```python
from build123d import *

# Parameters (mm, degrees)
CROQUIS1_R              = 10.5
SALIENTE_EXTRUIR1_DEPTH = 2.5
CROQUIS2_R              = 4.5
CROQUIS2_R_2            = 3
SALIENTE_EXTRUIR2_DEPTH = 3
CROQUIS4_R              = 4.75
CROQUIS4_R_2            = 3.25
CORTAR_EXTRUIR1_DEPTH   = 1
CROQUIS5_R              = 3
CORTAR_EXTRUIR2_DEPTH   = 1
CROQUIS6_R              = 1.5
CORTAR_EXTRUIR3_DEPTH   = 3
CROQUIS7_R              = 1
CORTAR_EXTRUIR4_DEPTH   = 3


with BuildPart() as part:
    # Croquis1 → Saliente-Extruir1 (new body)
    with BuildSketch(Plane(origin=(0, 0, 0), x_dir=(1, 0, 0), z_dir=(0, 1, 0))):
        with Locations(Location((0, 0, 0), (0, 0, 270))):
            Circle(CROQUIS1_R)
    extrude(amount=SALIENTE_EXTRUIR1_DEPTH)

    # Croquis2 → Saliente-Extruir2 (add)
    with BuildSketch(Plane(origin=(0, 2.5, 0), x_dir=(1, 0, 0), z_dir=(0, 1, 0))):
        with Locations(Location((0, 0, 0), (0, 0, 270))):
            Circle(CROQUIS2_R)
        with Locations(Location((0, 0, 0), (0, 0, 270))):
            Circle(CROQUIS2_R_2, mode=Mode.SUBTRACT)
    extrude(amount=SALIENTE_EXTRUIR2_DEPTH)

    # Croquis4 → Cortar-Extruir1 (cut)
    with BuildSketch(Plane.XZ):
        with Locations(Location((0, 0, 0), (0, 0, 270))):
            Circle(CROQUIS4_R)
        with Locations(Location((0, 0, 0), (0, 0, 270))):
            Circle(CROQUIS4_R_2, mode=Mode.SUBTRACT)
    extrude(amount=-CORTAR_EXTRUIR1_DEPTH, mode=Mode.SUBTRACT)

    # Croquis5 → Cortar-Extruir2 (cut)
    with BuildSketch(Plane.XZ):
        with Locations(Location((0, 0, 0), (0, 0, 90))):
            Circle(CROQUIS5_R)
    extrude(amount=-CORTAR_EXTRUIR2_DEPTH, mode=Mode.SUBTRACT)

    # Croquis6 → Cortar-Extruir3 (cut)
    with BuildSketch(Plane.XZ.offset(-1)):
        with Locations(Location((0, 0, 0), (0, 0, 270))):
            Circle(CROQUIS6_R)
    extrude(amount=-CORTAR_EXTRUIR3_DEPTH, mode=Mode.SUBTRACT)

    # Croquis7 → Cortar-Extruir4 (cut)
    with BuildSketch(Plane.XZ):
        with Locations(Location((0, 7.2, 0), (0, 0, 270))):
            Circle(CROQUIS7_R)
        with Locations(Location((0, -7.2, 0), (0, 0, 90))):
            Circle(CROQUIS7_R)
        with Locations(Location((7.2, 0, 0), (0, 0, 270))):
            Circle(CROQUIS7_R)
        with Locations(Location((-7.2, 0, 0), (0, 0, 90))):
            Circle(CROQUIS7_R)
        with Locations(Location((3.5, 7.2, 0), (0, 0, 270))):
            Circle(CROQUIS7_R)
        with Locations(Location((-3.5, 7.2, 0), (0, 0, 270))):
            Circle(CROQUIS7_R)
        with Locations(Location((3.5, -7.2, 0), (0, 0, 90))):
            Circle(CROQUIS7_R)
        with Locations(Location((-3.5, -7.2, 0), (0, 0, 90))):
            Circle(CROQUIS7_R)
        with Locations(Location((7.2, 3, 0), (0, 0, 270))):
            Circle(CROQUIS7_R)
        with Locations(Location((7.2, -3, 0), (0, 0, 270))):
            Circle(CROQUIS7_R)
        with Locations(Location((-7.2, -3, 0), (0, 0, 90))):
            Circle(CROQUIS7_R)
        with Locations(Location((-7.2, 3, 0), (0, 0, 90))):
            Circle(CROQUIS7_R)
    extrude(amount=-CORTAR_EXTRUIR4_DEPTH, mode=Mode.SUBTRACT)


solid = part.part
```
Read the model definition and answer for the solid it produces. Units are mm, in the model's axes. A direction names the side the tool comes from. Coordinates: 2 decimals unless noted, no trailing zeros. Write each loop counter-clockwise with the first axis right and the second up, starting at its lowest first coordinate (ties: lowest second). Pieces come first, ordered by that corner, then holes. Notation, with made-up numbers: (84, 49.25) -> (116, 49.25) arc R28 ccw to (116, 81.25) -> close; hole circle Ø1 at (28.25, 64.25). An arc over 180 degrees is marked (long way). Return JSON: item names as keys, results as strings.
1. A cutting plane is placed at A-A (y = 0.3). Give the number of separate pieces and of enclosed holes in the cut face, and give its area (3 significant figures).
Found:
{"separate pieces": "2", "enclosed holes": "14", "area": "243 mm2"}
2. Determine the mould class of faces 4 (the face through (-3, 1, -2)), 5 (the face through (-8.04, 1.23, 0.54)), 6 (the face through (3.2, 1.2, 10)), 7 (the face through (-2, 0, 5)) for opening direction X: pulls with the +X half, pulls with the -X half, needs draft (parallel to the pull), parting line crosses it, or undercut.
Found:
{"face 4": "undercut", "face 5": "undercut", "face 6": "parting line crosses it", "face 7": "needs draft"}
3. A cutting plane is placed at D-D (z = -7). Determine the outline of the cut face in (x, y).
Found:
{"outline": "(-7.83, 0) -> (-4.48, 0) -> (-4.48, 2.5) -> (-7.83, 2.5) -> close; (-2.52, 0) -> (-0.98, 0) -> (-0.98, 2.5) -> (-2.52, 2.5) -> close; (0.98, 0) -> (2.52, 0) -> (2.52, 2.5) -> (0.98, 2.5) -> close; (4.48, 0) -> (7.83, 0) -> (7.83, 2.5) -> (4.48, 2.5) -> close"}
4. Each of these flat-tipped pins is pushed along its axis until it touches: P1, Ø2.5, axis at x = 0, z = 0, coming from the +Y side; P2, Ø2.5, axis at x = -7.2, z = 3, coming from the +Y side; P3, Ø2, axis at y = 3, z = 7.5, coming from the +X side; P4, Ø1.8, axis at x = 0.5, z = 0.5, coming from the -Y side. Where does it stop, or does it pass through?
Found:
{"P1": "through", "P2": "y = 2.5", "P3": "x = 8.14", "P4": "y = 1"}
5. Find the intervals of material crossed by line 1 along X through (y, z) = (0.95, 0); line 2 along Z through (x, y) = (4, 0.65); line 3 along X through (y, z) = (0.5, 7.2), in increasing order. Write a range as from..to.
Found:
{"line 1": "-10.5..-8.2, -6.2..-4.75, -3.25..-3, 3..3.25, 4.75..6.2, 8.2..10.5", "line 2": "-9.71..-8.07, -6.33..-2.56, 2.56..6.33, 8.07..9.71", "line 3": "-7.64..-4.5, -2.5..-1, 1..2.5, 4.5..7.64"}
6. A tool of negligible diameter and unlimited length cuts with its end or side. For faces 1 (the face through (-1.3, 2.5, 1.3)), 2 (the face through (-0.383, 1.232, 6.276)), 3 (the face through (-1.978, 0.493, 2.579)), from which of +Z, -Z, +X, -X, +Y, -Y can it reach the whole face along a straight path? Write none if from no direction.
Found:
{"face 1": "+Y", "face 2": "+Y, -Y", "face 3": "-Y"}
